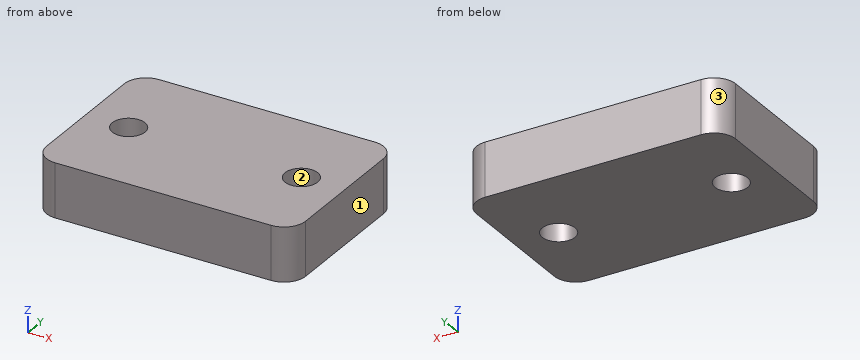
Autodesk Inventor part; units mm, degrees
ref_plane "YZ Plane" through (0, 0, 0) normal (1, 0, 0) x (0, 1, 0)
ref_plane "XZ Plane" through (0, 0, 0) normal (0, 1, 0) x (-1, 0, 0)
ref_plane "XY Plane" through (0, 0, 0) normal (0, 0, 1) x (1, 0, 0)
sketch "Sketch1" plane through (0, 0, 0) normal (0, 0, 1) x (1, 0, 0)
  line L0 (3.175, 0) -> (34.925, 0)
  line L1 (38.1, 3.175) -> (38.1, 22.225)
  line L2 (34.925, 25.4) -> (3.175, 25.4)
  line L3 (0, 22.225) -> (0, 3.175)
  circle A0 centre (6.35, 12.7) radius 2.413
  circle A1 centre (31.75, 12.7) radius 2.413
  line L4 (0, 12.7) -> (38.1, 12.7) construction
  arc A2 (3.175, 25.4) -> (0, 22.225) centre (3.175, 22.225) ccw
  arc A3 (38.1, 22.225) -> (34.925, 25.4) centre (34.925, 22.225) ccw
  arc A4 (34.925, 0) -> (38.1, 3.175) centre (34.925, 3.175) ccw
  arc A5 (0, 3.175) -> (3.175, 0) centre (3.175, 3.175) ccw
  point P0 (0, 0)
  point P1 (38.1, 25.4)
  point P2 (38.1, 0)
  point P3 (0, 25.4)
  dimension "d0" = 38.1
  dimension "d1" = 25.4
  dimension "d2" = 4.826
  dimension "d3" = 6.35
  dimension "d7" = 25.4
  dimension "d20" = 3.175
extrude "Extrusion1" add sketch "Sketch1" along normal blind 7.9375
properties part number "Bearing Mount Spacer 1-8in" material "ABS Plastic"
The listing builds one solid part. Answer for the finished solid, in the listing's coordinates (mm). Face numbers are marked on the shaded views. Give positions to 0.01 mm unless a question says otherwise; leave off trailing zeros. Order: outer loops, then holes, each group sorted by start corner. A loop starts at its lowest first (then second) coordinate and runs counter-clockwise, first axis right, second up. Notation, with made-up numbers: (76, 2.5) - (80, 2.5) arc R15 cw to (80, 17.5) - close; hole circle Ø6 at (77.25, 28). An arc over 180 degrees is marked (long way). One line per item, written item: value. Start each with the question number.
1) A cutting plane is placed at A-A on x = 6.35. Give the vertices of the cut face in (y, z), then the cut area to 3 significant figures.
2) A cutting plane is placed at D-D on x = 30.5. Give the vertices of the cut face in (y, z), then the cut area to 3 significant figures.
3) The mould has two halves that part along Y. Classify the marked faces 1, 2 and 3: released by +Y, released by -Y, zero draft, split by the parting line, or undercut.
4) A cutting plane is placed at B-B on y = 12.7. Give the vertices of the cut face in (x, z).
5) Given pin 1 Ø4 at (x, y) = (6.35, 12.7) entering from +Z, flat-ended and moving along its own axis, determine where the tip first touches the part or whether it passes through.
6) Find the intervals of material crossed by L1, parallel to Y at x = 31.75, z = 5.75; L2, parallel to X at y = 11.5, z = 4.5; L3, parallel to X at y = 14.5, z = 4, in increasing order.
7) A cutting plane is placed at C-C on z = 1. Give the vertices of the cut face in (x, y) (3 decimals).
Answer sheet:
1. outline: (0, 0) - (10.29, 0) - (10.29, 7.94) - (0, 7.94) - close; (15.11, 0) - (25.4, 0) - (25.4, 7.94) - (15.11, 7.94) - close
1. area: 163 mm2
2. outline: (0, 0) - (10.64, 0) - (10.64, 7.94) - (0, 7.94) - close; (14.76, 0) - (25.4, 0) - (25.4, 7.94) - (14.76, 7.94) - close
2. area: 169 mm2
3. face 1: zero draft
3. face 2: undercut
3. face 3: released by +Y
4. outline: (0, 0) - (3.94, 0) - (3.94, 7.94) - (0, 7.94) - close; (8.76, 0) - (29.34, 0) - (29.34, 7.94) - (8.76, 7.94) - close; (34.16, 0) - (38.1, 0) - (38.1, 7.94) - (34.16, 7.94) - close
5. pin 1: passes through
6. L1: y = 0 to 10.29, 15.11 to 25.4
6. L2: x = 0 to 4.26, 8.44 to 29.66, 33.84 to 38.1
6. L3: x = 0 to 4.74, 7.96 to 30.14, 33.36 to 38.1
7. outline: (0, 3.175) arc R3.175 ccw to (3.175, 0) - (34.925, 0) arc R3.175 ccw to (38.1, 3.175) - (38.1, 22.225) arc R3.175 ccw to (34.925, 25.4) - (3.175, 25.4) arc R3.175 ccw to (0, 22.225) - close; hole circle Ø4.826 at (6.35, 12.7); hole circle Ø4.826 at (31.75, 12.7)
